```python
from build123d import *

# Parameters (mm, degrees)
CHANFRO1_SIZE         = 0.8
FILETE1_R             = 2
ESBO_O2_W             = 2
ESBO_O2_H             = 30
CORTE_EXTRUS_O1_DEPTH = 3


with BuildPart() as part:
    # Esboço1 → Revolução1 (revolve)
    with BuildSketch(Plane.XY):
        Polygon((0, 0), (0, 12.5), (10, 12.5), (10, 3), (25, 3), (25, 0), align=None)
    revolve(axis=Axis((25, 0, 0), (-1, 0, 0)))

    # Chanfro1
    chanfro1_edges = [part.edges().sort_by_distance(p)[0] for p in [
        (25, -3, 0),
        (10, -12.5, 0),
        (0, -12.5, 0),
    ]]
    chamfer(chanfro1_edges, length=CHANFRO1_SIZE)

    # Filete1
    filete1_edges = [part.edges().sort_by_distance(p)[0] for p in [
        (10, -3, 0),
    ]]
    fillet(filete1_edges, radius=FILETE1_R)

    # Esboço2 → Corte-extrusão1 (cut)
    with BuildSketch(Plane.ZY):
        Rectangle(ESBO_O2_W, ESBO_O2_H)
    extrude(amount=-CORTE_EXTRUS_O1_DEPTH, mode=Mode.SUBTRACT)


solid = part.part
```
Geometry check sheet. Reference: the model listing, model coordinates, mm. A direction names the side the tool comes from. Round coordinates to 2 decimals unless told otherwise and drop trailing zeros. Order: outer loops, then holes, each group sorted by start corner. A loop starts at its lowest first (then second) coordinate and runs counter-clockwise, first axis right, second up. Notation, with made-up numbers: (43.5, 29) -> (68.5, 29) arc R20 cw to (68.5, 55) -> close; hole circle Ø11 at (46, 26). An arc over 180 degrees is marked (long way). Return JSON: item names as keys, results as strings. Group by question number.
Q1. Section check B-B, the plane z = 0. Record the boundary of the cut face in (x, y).
Q2. Section check A-A, the plane y = 0. Record the boundary of the cut face in (x, z).
Q3. Material ranges on probe 1 along X at (y, z) = (-3.25, 9.5); probe 2 along Y at (x, z) = (1.5, -4.5); probe 3 along Z at (x, y) = (1.5, 0.5), recorded low to high. Write a range as from..to.
Q4. Gauge pin test, flat ends, axial feed: pin 1 (4 mm diameter, centred on x = 18, y = -3.5, fed in from +Z); pin 2 (6 mm diameter, centred on x = 13.5, z = 1.5, fed in from +Y); pin 3 (6 mm diameter, centred on y = -1, z = 3.5, fed in from -X); pin 4 (10 mm diameter, centred on x = 4.5, y = 8.5, fed in from -Z). Record the tip position at first contact, or that the pin passes through.
Q5. Section check D-D, the plane x = 14. Record the boundary of the cut face in (y, z), plus the area to 3 significant figures.
Q6. Section check C-C, the plane x = 1.75. Record the boundary of the cut face in (y, z), plus the area to 3 significant figures.
Q7. Tool access check on faces 1 (the cylindrical face through (18, -3, 0)), 2 (the flat face through (0, 0, -5)), 3 (the flat face through (3, 0, 0)). Record the directions out of +Z, -Z, +X, -X, +Y, -Y that give a thin tool (end or side, any length) a straight path to the whole face; none if there is none.
Numbers:
{
 "1": {"outline": "(3, -12.5) -> (9.2, -12.5) -> (10, -11.7) -> (10, -5) arc R2 cw to (12, -3) -> (24.2, -3) -> (25, -2.2) -> (25, 2.2) -> (24.2, 3) -> (12, 3) arc R2 cw to (10, 5) -> (10, 11.7) -> (9.2, 12.5) -> (3, 12.5) -> close"},
 "2": {"outline": "(0, -11.7) -> (0.8, -12.5) -> (9.2, -12.5) -> (10, -11.7) -> (10, -5) arc R2 cw to (12, -3) -> (24.2, -3) -> (25, -2.2) -> (25, 2.2) -> (24.2, 3) -> (12, 3) arc R2 cw to (10, 5) -> (10, 11.7) -> (9.2, 12.5) -> (0.8, 12.5) -> (0, 11.7) -> (0, 1) -> (3, 1) -> (3, -1) -> (0, -1) -> close"},
 "3": {"probe 1": "0..10", "probe 2": "-11.66..11.66", "probe 3": "-12.49..-1, 1..12.49"},
 "4": {"pin 1": "z = 2.6", "pin 2": "y = 3.5", "pin 3": "x = 0", "pin 4": "z = -12"},
 "5": {"outline": "circle Ø6 at (0, 0)", "area": "28.3 mm^2"},
 "6": {"outline": "(-12.46, -1) arc R12.5 ccw to (12.46, -1) -> close; (-12.46, 1) -> (12.46, 1) arc R12.5 ccw to start", "area": "441 mm^2"},
 "7": {"face 1": "+X", "face 2": "+Z, -Z, -X, +Y, -Y", "face 3": "-X, +Y, -Y"}
}
